```python
from build123d import *

# Parameters (mm, degrees)
F0_W     = 100
F0_H     = 50
F0_W_2   = 600
F0_W_3   = 50
F0_W_4   = 775
F1_DEPTH = 3


with BuildPart() as f1:
    # F0 (on Front) → F1 (new body)
    with BuildSketch(Plane.XZ):
        with BuildLine():
            Line((-800, 92.0008493777), (-800, 0))
            Line((-800, 0), (-750, 0))
            Line((-750, 0), (-750, 50))
            Line((-750, 50), (-773.2805475772, 50))
            ThreePointArc((-773.2805475772, 50), (-786.7954423389, 70.9017119543), (-800.0000000001, 92.0008493776))
        make_face()
        with Locations((-700, 25)):
            Rectangle(F0_W, F0_H)
        with Locations((-350, 25)):
            Rectangle(F0_W_2, F0_H)
        with Locations((-25, 25)):
            Rectangle(F0_W_3, F0_H)
        with Locations((25, 25)):
            Rectangle(F0_W_3, F0_H)
        with Locations((350, 25)):
            Rectangle(F0_W_2, F0_H)
        with Locations((700, 25)):
            Rectangle(F0_W, F0_H)
        with BuildLine():
            Line((750, 0), (800, 0))
            Line((800, 0), (800, 92.0008493776))
            ThreePointArc((800.0000000001, 92.0008493776), (786.7954423389, 70.9017119543), (773.2805475772, 50))
            Line((773.2805475772, 50), (750, 50))
            Line((750, 50), (750, 0))
        make_face()
        with BuildLine():
            Line((-1049.2577214167, 925), (-1099.279129469, 925))
            ThreePointArc((-1099.279129469, 925), (-1015.7790507756, 441.1008996693), (-800, 0))
            Line((-800, 0), (-800, 92.0008493777))
            ThreePointArc((-800.0000000001, 92.0008493776), (-979.3055551093, 492.139557753), (-1049.2577214167, 925))
        make_face()
        with BuildLine():
            ThreePointArc((800, 0), (1015.7790507756, 441.1008996693), (1099.279129469, 925))
            Line((1099.279129469, 925), (1049.2577214167, 925))
            ThreePointArc((1049.2577214167, 925), (979.3055551094, 492.139557753), (800.0000000001, 92.0008493776))
            Line((800, 92.0008493776), (800, 0))
        make_face()
        with BuildLine():
            ThreePointArc((1099.279129469, 925), (1099.8197730031, 949.9974018634), (1100, 975))
            Line((1100, 975), (1050, 975))
            ThreePointArc((1050, 975), (1049.8144201308, 949.9972452643), (1049.2577214167, 925))
            Line((1049.2577214167, 925), (1099.279129469, 925))
        make_face()
        with BuildLine():
            Line((-1050, 975), (-1100, 975))
            ThreePointArc((-1100, 975), (-1099.8197730031, 949.9974018634), (-1099.279129469, 925))
            Line((-1099.279129469, 925), (-1049.2577214167, 925))
            ThreePointArc((-1049.2577214167, 925), (-1049.8144201308, 949.9972452643), (-1050, 975))
        make_face()
        with BuildLine():
            Line((-800, 925), (-1049.2577214167, 925))
            ThreePointArc((-1049.2577214167, 925), (-979.3055551093, 492.139557753), (-800.0000000001, 92.0008493776))
            Line((-800, 92.0008493777), (-800, 925))
        make_face()
        with BuildLine():
            Line((-25, 925), (-800, 925))
            Line((-800, 925), (-800, 92.0008493777))
            ThreePointArc((-800.0000000001, 92.0008493776), (-786.7954423389, 70.9017119543), (-773.2805475772, 50))
            Line((-773.2805475772, 50), (-750, 50))
            Line((-750, 50), (-650, 50))
            Line((-650, 50), (-50, 50))
            Line((-50, 50), (0, 50))
            Line((0, 50), (50, 50))
            Line((50, 50), (650, 50))
            Line((650, 50), (750, 50))
            Line((750, 50), (773.2805475772, 50))
            ThreePointArc((773.2805475772, 50), (786.7954423389, 70.9017119543), (800.0000000001, 92.0008493776))
            Line((800, 92.0008493776), (800, 925))
            Line((800, 925), (25, 925))
            Line((25, 925), (-25, 925))
        make_face()
        with BuildLine():
            ThreePointArc((800.0000000001, 92.0008493776), (979.3055551094, 492.139557753), (1049.2577214167, 925))
            Line((1049.2577214167, 925), (800, 925))
            Line((800, 925), (800, 92.0008493776))
        make_face()
        with BuildLine():
            ThreePointArc((1049.2577214167, 925), (1049.8144201308, 949.9972452643), (1050, 975))
            Line((1050, 975), (800, 975))
            Line((800, 975), (800, 925))
            Line((800, 925), (1049.2577214167, 925))
        make_face()
        with Locations((412.5, 950)):
            Rectangle(F0_W_4, F0_H)
        Polygon((25, 975), (0, 975), (-25, 975), (-25, 925), (25, 925), align=None)
        with Locations((-412.5, 950)):
            Rectangle(F0_W_4, F0_H)
        with BuildLine():
            Line((-800, 975), (-1050, 975))
            ThreePointArc((-1050, 975), (-1049.8144201308, 949.9972452643), (-1049.2577214167, 925))
            Line((-1049.2577214167, 925), (-800, 925))
            Line((-800, 925), (-800, 975))
        make_face()
    extrude(amount=F1_DEPTH)


solid = f1.part
```
The model under review builds one solid part; all positions refer to its coordinate system, in mm. Round coordinates to 2 decimals unless told otherwise and drop trailing zeros. Order: outer loops, then holes, each group sorted by start corner. A loop starts at its lowest first (then second) coordinate and runs counter-clockwise, first axis right, second up. Notation, with made-up numbers: (16, -27.75) -> (36, -27.75) arc R12 ccw to (36, -6.75) -> close; hole circle Ø10 at (-24, 1.5). An arc over 180 degrees is marked (long way). One line per item, written item: value. Start each with the question number.
Q1. Take a section at A-A (y = -0.95). Write out the cut boundary in (x, z) (3 decimals), and give its area (3 significant figures).
Q2. Wall thickness on line 1 (X direction, y = -0.6, z = 50); line 2 (X direction, y = -1.05, z = 628.5); line 3 (Z direction, x = -928, y = -2.1): over which ranges is each line inside the solid? List them lowest first.
Q3. Take a section at B-B (z = 63). Write out the cut boundary in (x, y), and give its area (3 significant figures).
Q4. Take a section at C-C (x = 919). Write out the cut boundary in (y, z).
Reported:
1. outline: (-1100, 975) arc R1734.375 ccw to (-800, 0) -> (800, 0) arc R1734.375 ccw to (1100, 975) -> close
1. area: 1,960,000 mm2
2. line 1: x = -832.74 to 832.74
2. line 2: x = -1065.04 to 1065.04
2. line 3: z = 221.98 to 975
3. outline: (-840.86, -3) -> (840.86, -3) -> (840.86, 0) -> (-840.86, 0) -> close
3. area: 5,050 mm2
4. outline: (-3, 203.58) -> (0, 203.58) -> (0, 975) -> (-3, 975) -> close
